The listing builds one solid part. Answer for the finished solid, in the listing's coordinates (mm). Give positions to 0.01 mm unless a question says otherwise; leave off trailing zeros. Write each loop counter-clockwise with the first axis right and the second up, starting at its lowest first coordinate (ties: lowest second). Pieces come first, ordered by that corner, then holes. Notation, with made-up numbers: (-39, 26.5) -> (3, 26.5) arc R17 ccw to (3, 57.5) -> close; hole circle Ø1 at (66, 57.25). An arc over 180 degrees is marked (long way). Write each question's results on one line, items separated by ' | '. Start each with the question number.
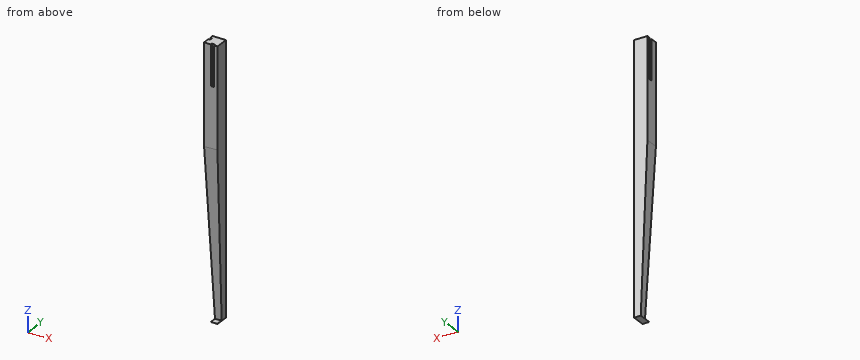
from build123d import *

# Parameters (mm, degrees)
F1_DEPTH = 50.8
F2_W     = 12.7
F2_H     = 152.4
F3_DEPTH = 6.35
F5_DEPTH = 65.988231
F6_W     = 12.7
F6_H     = 152.4
F7_DEPTH = 6.35


with BuildPart() as f1:
    # F0 (on Front) → F1 (new body)
    with BuildSketch(Plane.XZ):
        Polygon((0, -1016), (0, 0), (-50.8, 0), (-50.8, -381), (-25.4, -1016), align=None)
    extrude(amount=-F1_DEPTH)

    # F2 (on face) → F3 (cut)
    with BuildSketch(Plane(origin=(-50.8, 0, 0), x_dir=(0, -1, 0), z_dir=(-1, 0, 0))):
        with Locations((-31.75, -76.2)):
            Rectangle(F2_W, F2_H)
    extrude(amount=-F3_DEPTH, mode=Mode.SUBTRACT)

    # F4 (on face) → F5 (cut, through all)
    with BuildSketch(Plane(origin=(-65.934505, 0, -2.63738), x_dir=(0, -1, 0), z_dir=(-0.999201, 0, -0.039968))):
        Polygon((0, -1014.172986), (0, -378.665189), (-25.4, -1014.172986), align=None)
    extrude(amount=-F5_DEPTH, mode=Mode.SUBTRACT)

    # F6 (on face) → F7 (cut)
    with BuildSketch(Plane.XZ):
        with Locations((-19.05, -76.2)):
            Rectangle(F6_W, F6_H)
    extrude(amount=-F7_DEPTH, mode=Mode.SUBTRACT)


solid = f1.part
1. Section D-D (z = -665.5) is taken. Write down the section's boundary in (x, y).
2. Section B-B (x = -34) is taken. Write down the section's boundary in (y, z), then the cut area to 3 significant figures.
3. Section A-A (y = 16.5) is taken. Write down the section's boundary in (x, z).
4. Consider probe 1 along X at (y, z) = (5, -109); probe 2 along X at (y, z) = (46, -536); probe 3 along Y at (x, z) = (-24, -782). Determine where each line is inside the solid, lowest interval first. Write a range as [from, to].
5. Each of these flat-tipped pins is pushed along its axis until it touches: pin 1 Ø1.9 at (x, y) = (-46.5, 30) entering from +Z; pin 2 Ø2 at (x, y) = (-26, 19.5) entering from +Z; pin 3 Ø12 at (x, z) = (-37.5, -388.5) entering from -Y; pin 4 Ø8 at (x, z) = (-30, -734.5) entering from -Y. Where does it stop, or does it pass through?
6. Section C-C (z = -505.5) is taken. Write down the section's boundary in (x, y), then the cut area to 3 significant figures.
Results:
1) outline: (-39.42, 11.38) -> (0, 11.44) -> (0, 50.8) -> (-39.42, 50.8) -> close
2) outline: (0, -380.33) -> (16.8, -801) -> (50.8, -801) -> (50.8, 0) -> (0, 0) -> close | area: 37,200 mm²
3) outline: (-50.8, -381) -> (-34.3, -793.5) -> (0, -792.13) -> (0, 0) -> (-50.8, 0) -> close; (-25.4, -1016) -> (0, -1016) -> (0, -1014.98) -> close
4) probe 1: x = [-50.8, -25.4], [-12.7, 0] | probe 2: x = [-44.6, 0] | probe 3: y = [16.06, 50.8]
5) pin 1: stops at z = -152.4 | pin 2: stops at z = 0 | pin 3: stops at y = 0.08 | pin 4: stops at y = 13.99
6) outline: (-45.82, 4.98) -> (0, 5.05) -> (0, 50.8) -> (-45.82, 50.8) -> close | area: 2,100 mm²
